Input: part model. Units: mm. Frame: model coordinates. A direction names the side the tool comes from. Coordinates: 2 decimals unless noted, no trailing zeros. Order: outer loops, then holes, each group sorted by start corner. A loop starts at its lowest first (then second) coordinate and runs counter-clockwise, first axis right, second up. Notation, with made-up numbers: (65.25, -17) - (93.25, -17) arc R23 ccw to (93.25, 19) - close; hole circle Ø4 at (80, 54.25). An arc over 180 degrees is marked (long way). Answer as CSV lines item,"result". Start each with the question number.
Item 1: Access query for faces 1 (the flat face through (10, 2, 0)), 2 (the flat face through (10, -35, 30.923)), 3 (the cylindrical face through (7.82, -22.08, 30.05)), 4 (the flat face through (10, -35, -30.923)). Directions: +Z, -Z, +X, -X, +Y, -Y. A direction counts if a zero-diameter tool reaches every point of the face in a straight line with its end or side. Return the directions, or none.
Item 2: Section C-C (y = -18). Output: boundary loops of the cut face in (x, z).
Item 3: Section A-A (x = 17.5). Output: boundary loops of the cut face in (y, z) (3 decimals).
Item 4: Draft query along Z for faces 5 (the flat face through (17, -29.5, 0)), 6 (the cylindrical face through (17.362, -31.004, 29.497)), 7 (the cylindrical face through (5.1, 22.6, -19.1)). Return one class per face: +Z half, -Z half, draft (parallel to the pull), parting line (faces both ways), or undercut.
Item 5: First-contact query: pin 1 (3 mm diameter, centred on x = 18, z = -9.5, fed in from +Y); pin 2 (8 mm diameter, centred on y = 19.5, z = 19.5, fed in from +X). Flat tips, straight axial feed; report the tip coordinate or a pass-through.
Item 6: Section B-B (z = -18). Output: boundary loops of the cut face in (x, y) (3 decimals), and give its area (3 significant figures).
Item 7: Section D-D (z = 0). Output: boundary loops of the cut face in (x, y).
Item 8: Material intervals for line 1 along Z through (x, y) = (8.5, -20); line 2 along X through (y, z) = (-38.75, 18) (3 decimals); line 3 along Z through (x, y) = (18.75, -40), sorted ascending.
from build123d import *

# Parameters (mm, degrees)
SKETCH1_R           = 32.5
BOSS_EXTRUDE1_DEPTH = 10
SKETCH2_R           = 3.125
CUT_EXTRUDE1_DEPTH  = 11
BOSS_EXTRUDE2_DEPTH = 10
SKETCH4_W           = 61.846584384
SKETCH4_H           = 15
BOSS_EXTRUDE3_DEPTH = 15
SKETCH5_R           = 2.475
CUT_EXTRUDE2_DEPTH  = 16
FILLET1_R           = 5


with BuildPart() as part:
    # Sketch1 → Boss-Extrude1 (new body)
    with BuildSketch(Plane(origin=(0, 0, 0), x_dir=(0, 0, -1), z_dir=(1, 0, 0))):
        Circle(SKETCH1_R)
    extrude(amount=BOSS_EXTRUDE1_DEPTH)

    # Sketch2 → Cut-Extrude1 (cut, through all)
    with BuildSketch(Plane(origin=(10, 0, 0), x_dir=(0, 0, -1), z_dir=(1, 0, 0))):
        with Locations((-19.502005025, -19.502005025)):
            Circle(SKETCH2_R)
        with Locations((-19.502005025, 19.502005025)):
            Circle(SKETCH2_R)
        with Locations((19.502005025, 19.502005025)):
            Circle(SKETCH2_R)
        with Locations((19.502005025, -19.502005025)):
            Circle(SKETCH2_R)
    extrude(amount=-CUT_EXTRUDE1_DEPTH, mode=Mode.SUBTRACT)



with BuildPart() as body_2:
    # Sketch3 → Boss-Extrude2 (new body)
    with BuildSketch(Plane.ZY):
        with BuildLine():
            Line((-30.923292192, -10), (-30.923292192, -44.5))
            Line((-30.923292192, -44.5), (30.923292192, -44.5))
            Line((30.923292192, -44.5), (30.923292192, -10))
            ThreePointArc((30.923292192, -10), (0, -32.5), (-30.923292192, -10))
        make_face()
    extrude(amount=-BOSS_EXTRUDE2_DEPTH)


with BuildPart() as part_1:
    add(part.part)

    add(body_2.part)  # Boss-Extrude3 merges body 2
    # Sketch4 → Boss-Extrude3 (add)
    with BuildSketch(Plane(origin=(10, 0, 0), x_dir=(0, 0, -1), z_dir=(1, 0, 0))):
        with Locations((0, -37)):
            Rectangle(SKETCH4_W, SKETCH4_H)
    extrude(amount=BOSS_EXTRUDE3_DEPTH)

    # Sketch5 → Cut-Extrude2 (cut, through all)
    with BuildSketch(Plane(origin=(0, -29.5, 0), x_dir=(1, 0, 0), z_dir=(0, 1, 0))):
        with Locations((17.5, -18)):
            Circle(SKETCH5_R)
        with Locations((17.5, 18)):
            Circle(SKETCH5_R)
    extrude(amount=-CUT_EXTRUDE2_DEPTH, mode=Mode.SUBTRACT)

    # Fillet1
    fillet1_edges = [part_1.edges().sort_by_distance(p)[0] for p in [
        (17.5, -29.5, 30.923292192),
        (17.5, -29.5, -30.923292192),
        (10, -19.75, -30.923292192),
        (10, -19.75, 30.923292192),
    ]]
    fillet(fillet1_edges, radius=FILLET1_R)


solid = part_1.part
Determined:
1,face 1,"+Z, -Z, +X, +Y"
1,face 2,"+Z, +X, -X, -Y"
1,face 3,"+Z, +X"
1,face 4,"-Z, +X, -X, -Y"
2,outline,"(0, -30.92) - (5, -30.92) arc R5 ccw to (9.87, -27.06) - (10, -27.06) - (10, -22.24) - (0, -22.24) - close; (0, -16.76) - (10, -16.76) - (10, 16.76) - (0, 16.76) - close; (0, 22.24) - (10, 22.24) - (10, 27.06) - (9.87, 27.06) arc R5 ccw to (5, 30.92) - (0, 30.92) - close"
3,outline,"(-44.5, -30.923) - (-34.5, -30.923) arc R5 ccw to (-29.5, -25.923) - (-29.5, -20.475) - (-44.5, -20.475) - close; (-44.5, -15.525) - (-29.5, -15.525) - (-29.5, 15.525) - (-44.5, 15.525) - close; (-44.5, 20.475) - (-29.5, 20.475) - (-29.5, 25.923) arc R5 ccw to (-34.5, 30.923) - (-44.5, 30.923) - close"
4,face 5,"draft"
4,face 6,"+Z half"
4,face 7,"undercut"
5,pin 1,"stops at y = -29.5"
5,pin 2,"stops at x = 10"
6,outline,"(0, -44.5) - (15.025, -44.5) - (15.025, -29.5) - (10, -29.5) - (10, -22.242) - (0, -22.242) - close; (0, -16.762) - (10, -16.762) - (10, 16.762) - (0, 16.762) - close; (0, 22.242) - (10, 22.242) - (10, 27.06) - (0, 27.06) - close; (19.975, -44.5) - (25, -44.5) - (25, -29.5) - (19.975, -29.5) - close"
6,area,"757 mm^2"
7,outline,"(0, -44.5) - (25, -44.5) - (25, -29.5) - (10, -29.5) - (10, 32.5) - (0, 32.5) - close"
8,line 1,"z = -29.49 to -22.59, -16.42 to 16.42, 22.59 to 29.49"
8,line 2,"x = 0 to 15.025, 19.975 to 25"
8,line 3,"z = -30.92 to -20.14, -15.86 to 15.86, 20.14 to 30.92"
